Work out the finished part from the listing and answer in its coordinate system (mm). A direction names the side the tool comes from. Round coordinates to 2 decimals unless told otherwise and drop trailing zeros. Order: outer loops, then holes, each group sorted by start corner. A loop starts at its lowest first (then second) coordinate and runs counter-clockwise, first axis right, second up. Notation, with made-up numbers: (47, 82) - (65, 82) arc R30 ccw to (65, 121) - close; hole circle Ø11 at (27.25, -15). An arc over 180 degrees is marked (long way). Use one line per item in the form item = value. Start each with the question number.
Q1. For a pull along Z with two mould halves and no side action, classify faces 1 (the flat face through (0, 1, -20)), 2 (the flat face through (10, 5, 10)), 3 (the cylindrical face through (-7.767, 3.986, 9.49)), 4 (the cylindrical face through (11.733, 3.986, 9.49)) as +Z half, -Z half, draft (parallel to the pull), parting line (faces both ways), or undercut.
Q2. Which of the six approach directions +Z, -Z, +X, -X, +Y, -Y give full straight-line access (tool end or side, diameter ignored) to faces 5 (the cylindrical face through (11.733, 3.986, -10.01)), 6 (the cylindrical face through (15.313, 1.479, -17.223))?
Q3. Given P1, Ø1, axis at x = -3, z = 11, coming from the +Y side; P2, Ø2.5, axis at x = -15.22, z = -15.22, coming from the -Y side, each flat-ended and moving along its own axis, determine where each tip first touches the part or whether it passes through.
Q4. The part is cut by section C-C on y = 0.85. Determine the outline of the cut face in (x, z), plus the area to 3 significant figures.
Q5. The part is cut by section A-A on x = -9.75. Determine the outline of the cut face in (y, z).
Q6. The part is cut by section B-B on z = 9.75. Determine the outline of the cut face in (x, y), plus the area to 3 significant figures.
Q7. Find the intervals of material crossed by line 1 (X direction, y = 0.8, z = -16.5); line 2 (Y direction, x = -1, z = 14.5); line 3 (X direction, y = 4.2, z = -9.5), in increasing order. Write a range as [from, to].
Q8. The part is cut by section D-D on z = -16.5. Determine the outline of the cut face in (x, y).
from build123d import *

# Parameters (mm, degrees)
SKETCH_2_W          = 40
SKETCH_2_H          = 40
EXTRUDE_2_DEPTH     = 3
SKETCH_3_R          = 2
CUT_EXTRUDE_1_DEPTH = 3
SKETCH_2_6_R        = 2
EXTRUDE_3_DEPTH     = 5


with BuildPart() as part:
    # Sketch 2 → Extrude 2 (new body)
    with BuildSketch(Plane(origin=(0, 0, 0), x_dir=(1, 0, 0), z_dir=(0, 1, 0))):
        Rectangle(SKETCH_2_W, SKETCH_2_H)
    extrude(amount=EXTRUDE_2_DEPTH)

    # Sketch 3 → Cut-Extrude 1 (cut)
    with BuildSketch(Plane(origin=(0, 0, 0), x_dir=(1, 0, 0), z_dir=(0, 1, 0))):
        with Locations(Location((-15.224798987, -15.224798987, 0), (0, 0, 270))):
            Circle(SKETCH_3_R)
        with Locations(Location((15.224798987, -15.224798987, 0), (0, 0, 270))):
            Circle(SKETCH_3_R)
        with Locations(Location((15.224798987, 15.224798987, 0), (0, 0, 270))):
            Circle(SKETCH_3_R)
        with Locations(Location((-15.224798987, 15.224798987, 0), (0, 0, 270))):
            Circle(SKETCH_3_R)
    extrude(amount=CUT_EXTRUDE_1_DEPTH, mode=Mode.SUBTRACT)

    # Sketch 2_6 → Extrude 3 (add)
    with BuildSketch(Plane(origin=(0, 0, 0), x_dir=(1, 0, 0), z_dir=(0, 1, 0))):
        with Locations(Location((9.75, 9.75, 0), (0, 0, 270))):
            Circle(SKETCH_2_6_R)
        with Locations(Location((-9.75, 9.75, 0), (0, 0, 270))):
            Circle(SKETCH_2_6_R)
        with Locations(Location((9.75, -9.75, 0), (0, 0, 270))):
            Circle(SKETCH_2_6_R)
        with Locations(Location((-9.75, -9.75, 0), (0, 0, 270))):
            Circle(SKETCH_2_6_R)
    extrude(amount=EXTRUDE_3_DEPTH)


solid = part.part
Found:
q1.face_1 = -Z half
q1.face_2 = draft
q1.face_3 = undercut
q1.face_4 = undercut
q2.face_5 = +Y
q2.face_6 = +Y, -Y
q3.P1 = 3
q3.P2 = through
q4.outline = (-20, -20) - (20, -20) - (20, 20) - (-20, 20) - close; hole circle Ø4 at (-15.22, -15.22); hole circle Ø4 at (-15.22, 15.22); hole circle Ø4 at (15.22, -15.22); hole circle Ø4 at (15.22, 15.22)
q4.area = 1,550 mm²
q5.outline = (0, -20) - (3, -20) - (3, -11.75) - (5, -11.75) - (5, -7.75) - (3, -7.75) - (3, 7.75) - (5, 7.75) - (5, 11.75) - (3, 11.75) - (3, 20) - (0, 20) - close
q6.outline = (-20, 0) - (20, 0) - (20, 3) - (11.75, 3) - (11.75, 5) - (7.75, 5) - (7.75, 3) - (-7.75, 3) - (-7.75, 5) - (-11.75, 5) - (-11.75, 3) - (-20, 3) - close
q6.area = 136 mm²
q7.line_1 = [-20, -16.77], [-13.68, 13.68], [16.77, 20]
q7.line_2 = [0, 3]
q7.line_3 = [-11.73, -7.77], [7.77, 11.73]
q8.outline = (-20, 0) - (-16.77, 0) - (-16.77, 3) - (-20, 3) - close; (-13.68, 0) - (13.68, 0) - (13.68, 3) - (-13.68, 3) - close; (16.77, 0) - (20, 0) - (20, 3) - (16.77, 3) - close
